from build123d import *

# Parameters (mm, degrees)
SKETCH1_W           = 200
SKETCH1_H           = 80
BOSS_EXTRUDE1_DEPTH = 3
SKETCH2_R           = 2
CUT_EXTRUDE1_DEPTH  = 108.745069493
FILLET1_R           = 10
SKETCH3_R           = 1.5621
CUT_EXTRUDE2_DEPTH  = 108.745069493
SKETCH4_W           = 20
SKETCH4_H           = 20
CUT_EXTRUDE3_DEPTH  = 108.745069493
FILLET2_R           = 5
CUT_EXTRUDE4_DEPTH  = 108.745069493


with BuildPart() as part:
    # Sketch1 → Boss-Extrude1 (new body)
    with BuildSketch(Plane.XY):
        Rectangle(SKETCH1_W, SKETCH1_H)
    extrude(amount=BOSS_EXTRUDE1_DEPTH)

    # Sketch2 → Cut-Extrude1 (cut, through all)
    with BuildSketch(Plane.XY.offset(3)):
        with Locations((-92, 32)):
            Circle(SKETCH2_R)
        with Locations(Location((-92, -32, 0), (0, 0, 180))):
            Circle(SKETCH2_R)
        with Locations((92, -32)):
            Circle(SKETCH2_R)
        with Locations(Location((92, 32, 0), (0, 0, 180))):
            Circle(SKETCH2_R)
    extrude(amount=-CUT_EXTRUDE1_DEPTH, mode=Mode.SUBTRACT)

    # Fillet1
    fillet1_edges = [part.edges().sort_by_distance(p)[0] for p in [
        (100, -40, 1.5),
        (-100, -40, 1.5),
        (-100, 40, 1.5),
        (100, 40, 1.5),
    ]]
    fillet(fillet1_edges, radius=FILLET1_R)

    # Sketch3 → Cut-Extrude2 (cut, through all)
    with BuildSketch(Plane.XY.offset(3)):
        with Locations((36.6776, 24.1681)):
            Circle(SKETCH3_R)
        with Locations((36.6776, -24.1681)):
            Circle(SKETCH3_R)
        with Locations((-38.4556, -24.1681)):
            Circle(SKETCH3_R)
        with Locations((-45.9486, 24.1681)):
            Circle(SKETCH3_R)
        with Locations((-14.9479, 19.289607234)):
            Circle(SKETCH3_R)
    extrude(amount=-CUT_EXTRUDE2_DEPTH, mode=Mode.SUBTRACT)

    # Sketch4 → Cut-Extrude3 (cut, through all)
    with BuildSketch(Plane.XY.offset(3)):
        with Locations((80, 0)):
            Rectangle(SKETCH4_W, SKETCH4_H)
    extrude(amount=-CUT_EXTRUDE3_DEPTH, mode=Mode.SUBTRACT)

    # Fillet2
    fillet2_edges = [part.edges().sort_by_distance(p)[0] for p in [
        (90, 10, 1.5),
        (90, -10, 1.5),
        (70, -10, 1.5),
        (70, 10, 1.5),
    ]]
    fillet(fillet2_edges, radius=FILLET2_R)

    # Sketch5 → Cut-Extrude4 (cut, through all)
    with BuildSketch(Plane.XY.offset(3)):
        with BuildLine():
            Line((-15, -30), (15, -30))
            ThreePointArc((15, -30), (18, -33), (15, -36))
            Line((15, -36), (-15, -36))
            ThreePointArc((-15, -36), (-18, -33), (-15, -30))
        make_face()
        with BuildLine():
            Line((-15, 30), (15, 30))
            ThreePointArc((15, 30), (18, 33), (15, 36))
            Line((15, 36), (-15, 36))
            ThreePointArc((-15, 36), (-18, 33), (-15, 30))
        make_face()
    extrude(amount=-CUT_EXTRUDE4_DEPTH, mode=Mode.SUBTRACT)


solid = part.part
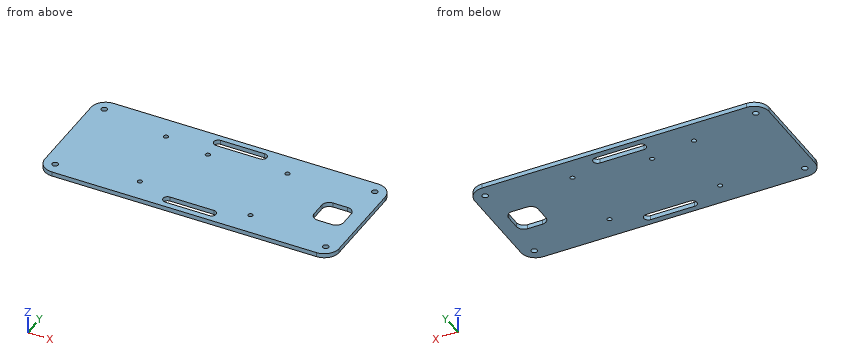
Geometry: final body of the model. Coordinates: model frame, mm. Round coordinates to 2 decimals unless told otherwise and drop trailing zeros. Loops run counter-clockwise (first coordinate to the right, second up) from the corner with the lowest first, then second, coordinate; pieces in that order, holes last. Notation, with made-up numbers: (73.25, 37) -> (101.25, 37) arc R25 ccw to (101.25, 63) -> close; hole circle Ø11 at (-24.5, 49.25). An arc over 180 degrees is marked (long way). One line per question, with ' | ' between items. Start each with the question number.
1. Section B-B on x = 10.5. Output: boundary loops of the cut face in (y, z).
2. Section D-D on z = 1.95. Count the separate pieces of the cut face and the enclosed holes in it, and give its area (3 significant figures).
3. Contact query for a flat-ended pin moving along its axis: pin 1 (2.5 mm diameter, centred on x = -38.46, y = -24.17, fed in from -Z). Output: stop coordinate, or through.
4. Section C-C on y = -32. Output: boundary loops of the cut face in (x, z).
5. Line query: line 1 along Y through (x, z) = (15.5, 2.4); line 2 along X through (y, z) = (1.5, 2.6); line 3 along Y through (x, z) = (37.5, 0.9). Output: solid intervals per line, ascending. Write a range as [from, to].
6. Section A-A on y = 2.5. Output: boundary loops of the cut face in (x, z).
Returned:
1) outline: (-40, 0) -> (-36, 0) -> (-36, 3) -> (-40, 3) -> close; (-30, 0) -> (30, 0) -> (30, 3) -> (-30, 3) -> close; (36, 0) -> (40, 0) -> (40, 3) -> (36, 3) -> close
2) separate pieces: 1 | enclosed holes: 12 | area: 15,000 mm2
3) pin 1: passes through
4) outline: (-99.8, 0) -> (-94, 0) -> (-94, 3) -> (-99.8, 3) -> close; (-90, 0) -> (-17.83, 0) -> (-17.83, 3) -> (-90, 3) -> close; (17.83, 0) -> (90, 0) -> (90, 3) -> (17.83, 3) -> close; (94, 0) -> (99.8, 0) -> (99.8, 3) -> (94, 3) -> close
5) line 1: y = [-40, -35.96], [-30.04, 30.04], [35.96, 40] | line 2: x = [-100, 70], [90, 100] | line 3: y = [-40, -25.5], [-22.84, 22.84], [25.5, 40]
6) outline: (-100, 0) -> (70, 0) -> (70, 3) -> (-100, 3) -> close; (90, 0) -> (100, 0) -> (100, 3) -> (90, 3) -> close
